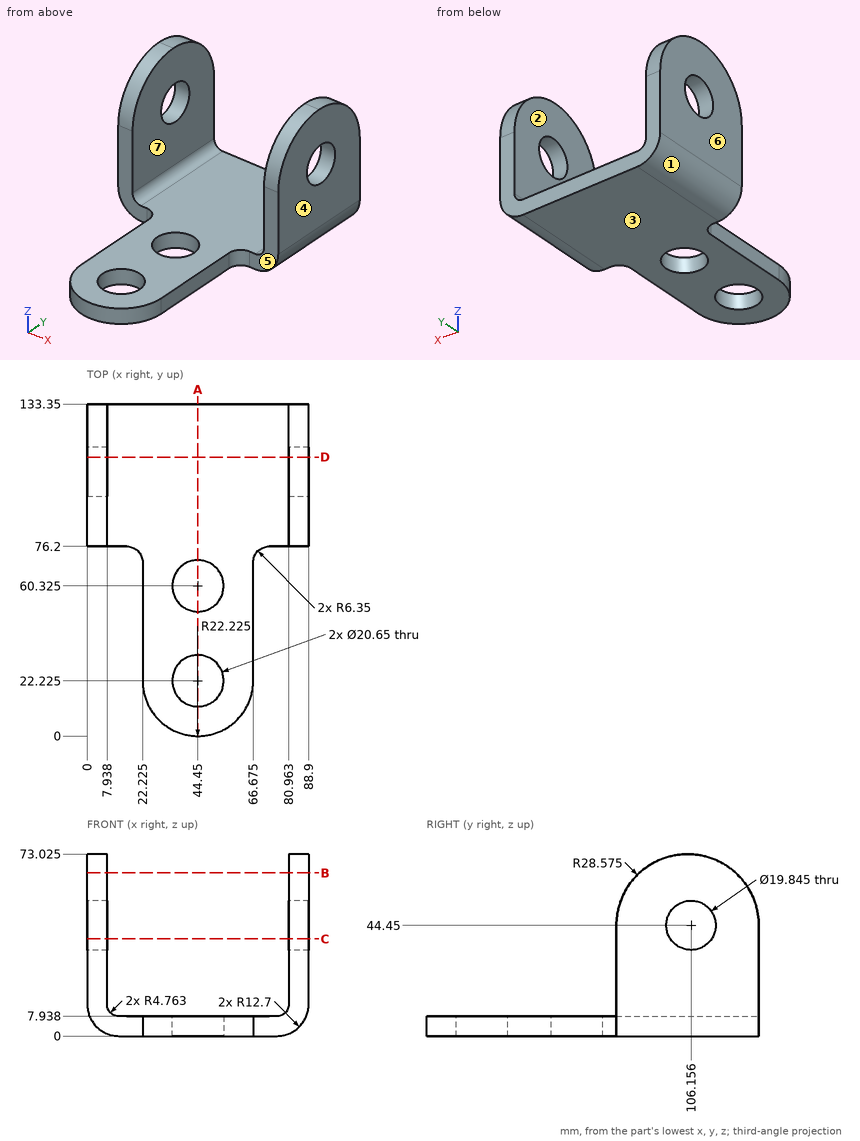
Could you check a few things on this drawing? It's one solid part, dimensions in mm from its lowest x, y, z. A direction names the side the tool comes from. Round coordinates to 2 decimals unless told otherwise and drop trailing zeros. Order: outer loops, then holes, each group sorted by start corner. A loop starts at its lowest first (then second) coordinate and runs counter-clockwise, first axis right, second up.
(1) Imagine slicing it at A-A (x = 44.45). Write out the boundary of the cut face in (y, z).
Response values:
outline: (0, 0) - (11.9, 0) - (11.9, 7.94) - (0, 7.94) - close; (32.55, 0) - (50, 0) - (50, 7.94) - (32.55, 7.94) - close; (70.65, 0) - (133.35, 0) - (133.35, 7.94) - (70.65, 7.94) - close
(2) Which directions (+Z, -Z, +X, -X, +Y, -Y) give clear straight access to the entire face, cutting with the end or side of a thin tool? Please do the marked faces 5, 6 and 7.
Response values:
face 5: +Z, -Z, +X, -Y
face 6: +Z, -Z, -X, +Y, -Y
face 7: +Z, +Y, -Y
(3) Please list where these lines run through material, in increasing order: line 1 along Y through (x, z) = (44.45, 3.25); line 2 along X through (y, z) = (96.5, 38); line 3 along Z through (x, y) = (34.5, 18).
Response values:
line 1: y = 0 to 11.9, 32.55 to 50, 70.65 to 133.35
line 2: x = 0 to 7.94, 80.96 to 88.9
line 3: z = 0 to 7.94
(4) If we mould it in two halves opening along X, with no side actions, what happens to the marked faces 1, 2, 3 and 4? For each: released by +X, released by -X, zero draft, split by the parting line, or undercut.
Response values:
face 1: released by -X
face 2: undercut
face 3: zero draft
face 4: released by +X
(5) Imagine slicing it at D-D (y = 112). Write out the boundary of the cut face in (x, z) (1 decimal), plus the area to 3 significant figures.
Response values:
outline: (0, 12.7) arc R12.7 ccw to (12.7, 0) - (76.2, 0) arc R12.7 ccw to (88.9, 12.7) - (88.9, 36.4) - (81, 36.4) - (81, 12.7) arc R4.8 cw to (76.2, 7.9) - (12.7, 7.9) arc R4.8 cw to (7.9, 12.7) - (7.9, 36.4) - (0, 36.4) - close; (0, 52.5) - (7.9, 52.5) - (7.9, 72.1) - (0, 72.1) - close; (81, 52.5) - (88.9, 52.5) - (88.9, 72.1) - (81, 72.1) - close
area: 1,410 mm2
(6) Imagine slicing it at B-B (z = 65.5). Write out the boundary of the cut face in (x, y).
Response values:
outline: (0, 85.45) - (7.94, 85.45) - (7.94, 124.1) - (0, 124.1) - close; (80.96, 85.45) - (88.9, 85.45) - (88.9, 124.1) - (80.96, 124.1) - close
(7) Imagine slicing it at C-C (z = 39). Count the separate pieces of the cut face and the enclosed holes in it, plus the area to 3 significant figures.
Response values:
separate pieces: 4
enclosed holes: 0
area: 644 mm2
(8) I'm going to push flat-ended pins straight in: pin 1 (17 mm diameter, centred on y = 98.5, z = 41, fed in from +X); pin 2 (4 mm diameter, centred on y = 55, z = 3.5, fed in from -X) (1 decimal); pin 3 (8.5 mm diameter, centred on y = 39, z = 3, fed in from +X) (1 decimal); pin 4 (4 mm diameter, centred on x = 51.5, y = 92.5, fed in from +Z). Where does each tip first touch, or does it pass through?
Response values:
pin 1: stops at x = 88.9
pin 2: stops at x = 22.2
pin 3: stops at x = 66.7
pin 4: stops at z = 7.94
